Here's how the part is built. I have some questions about the finished solid (model axes, mm). A direction names the side the tool comes from. Coordinates: 2 decimals unless noted, no trailing zeros. Write each loop counter-clockwise with the first axis right and the second up, starting at its lowest first coordinate (ties: lowest second). Pieces come first, ordered by that corner, then holes. Notation, with made-up numbers: M -35,-27.5 L -14,-27.5 A25 ccw -14,3.5 Z; hole C 15.25,9.25 d8. An arc over 180 degrees is marked long. Use a Markdown table: item, result.
```python
from build123d import *

# Parameters (mm, degrees)
SKETCH1_W               = 111.06
SKETCH1_H               = 59.85
FACE_2_DEPTH            = 3.86
FACE_FILLETS_R          = 1
SKETCH2_W               = 106.25
SKETCH2_H               = 55.5
BODY_DEPTH              = 144
SKETCH3_W               = 12.75
SKETCH3_H               = 12.75
FEET_DEPTH              = 3.33
FEET_DRAFT              = 25
FEET_PROFILE_2_DEPTH    = 3.33
FEET_PROFILE_2_DRAFT    = 25
FEET_PROFILE_3_DEPTH    = 3.33
FEET_PROFILE_3_DRAFT    = 25
FEET_PROFILE_4_DEPTH    = 3.33
FEET_PROFILE_4_DRAFT    = 25
BODY_FILLETS_R          = 1
SKETCH4_R               = 5
GND_BANNANA_PORT_DEPTH  = 5.15
FILLET3_R               = 1
SKETCH5_W               = 50.3
SKETCH5_H               = 30.9
POWER_PORT_DEPTH        = 3.5
FILLET4_R               = 1
BOSS_EXTRUDE6_DEPTH     = 8.1
SKETCH7_R               = 6.5
BOSS_EXTRUDE7_DEPTH     = 2.35
SKETCH8_R               = 2.65
BOSS_EXTRUDE8_DEPTH     = 0.3
MIRROR2_COPY_1_SKETCH_R = 2.65
MIRROR2_COPY_1_DEPTH    = 0.3


with BuildPart() as part:
    # Sketch1 → Face 2 (new body)
    with BuildSketch(Plane.XY):
        Rectangle(SKETCH1_W, SKETCH1_H)
    extrude(amount=FACE_2_DEPTH)

    # Face Fillets
    face_fillets_edges = [part.edges().sort_by_distance(p)[0] for p in [
        (55.53, -29.925, 1.93),
        (-55.53, -29.925, 1.93),
        (-55.53, 29.925, 1.93),
        (55.53, 29.925, 1.93),
    ]]
    fillet(face_fillets_edges, radius=FACE_FILLETS_R)

    # Sketch2 → Body (add)
    with BuildSketch(Plane.XY):
        Rectangle(SKETCH2_W, SKETCH2_H)
    extrude(amount=BODY_DEPTH)


with BuildPart() as feet_tool:
    # Sketch3 → Feet (with draft: the straight prism first)
    with BuildSketch(Plane.XZ.offset(27.75)):
        with Locations((-36.625, 125.75)):
            Rectangle(SKETCH3_W, SKETCH3_H)
    extrude(amount=FEET_DEPTH)
    # Feet: the draft: its side faces are tilted about the plane it starts from
    feet_sides = [feet_tool.faces().sort_by_distance(p)[0] for p in [
        (-36.625, -29.415, 119.375),
        (-30.25, -29.415, 125.75),
        (-36.625, -29.415, 132.125),
        (-43, -29.415, 125.75),
    ]]
    draft(feet_sides, Plane.XZ.offset(27.75), FEET_DRAFT)


with BuildPart() as part_1:
    add(part.part)

    # Feet: add feet_tool
    add(feet_tool.part)


with BuildPart() as feet_profile_2_tool:
    # Sketch3 → Feet profile 2 (with draft: the straight prism first)
    with BuildSketch(Plane.XZ.offset(27.75)):
        with Locations((36.625, 125.75)):
            Rectangle(SKETCH3_W, SKETCH3_H)
    extrude(amount=FEET_PROFILE_2_DEPTH)
    # Feet profile 2: the draft: its side faces are tilted about the plane it starts from
    feet_profile_2_sides = [feet_profile_2_tool.faces().sort_by_distance(p)[0] for p in [
        (36.625, -29.415, 119.375),
        (43, -29.415, 125.75),
        (36.625, -29.415, 132.125),
        (30.25, -29.415, 125.75),
    ]]
    draft(feet_profile_2_sides, Plane.XZ.offset(27.75), FEET_PROFILE_2_DRAFT)


with BuildPart() as part_2:
    add(part_1.part)

    # Feet profile 2: add feet_profile_2_tool
    add(feet_profile_2_tool.part)


with BuildPart() as feet_profile_3_tool:
    # Sketch3 → Feet profile 3 (with draft: the straight prism first)
    with BuildSketch(Plane.XZ.offset(27.75)):
        with Locations((36.625, 18.86)):
            Rectangle(SKETCH3_W, SKETCH3_H)
    extrude(amount=FEET_PROFILE_3_DEPTH)
    # Feet profile 3: the draft: its side faces are tilted about the plane it starts from
    feet_profile_3_sides = [feet_profile_3_tool.faces().sort_by_distance(p)[0] for p in [
        (36.625, -29.415, 12.485),
        (43, -29.415, 18.86),
        (36.625, -29.415, 25.235),
        (30.25, -29.415, 18.86),
    ]]
    draft(feet_profile_3_sides, Plane.XZ.offset(27.75), FEET_PROFILE_3_DRAFT)


with BuildPart() as part_3:
    add(part_2.part)

    # Feet profile 3: add feet_profile_3_tool
    add(feet_profile_3_tool.part)


with BuildPart() as feet_profile_4_tool:
    # Sketch3 → Feet profile 4 (with draft: the straight prism first)
    with BuildSketch(Plane.XZ.offset(27.75)):
        with Locations((-36.625, 18.86)):
            Rectangle(SKETCH3_W, SKETCH3_H)
    extrude(amount=FEET_PROFILE_4_DEPTH)
    # Feet profile 4: the draft: its side faces are tilted about the plane it starts from
    feet_profile_4_sides = [feet_profile_4_tool.faces().sort_by_distance(p)[0] for p in [
        (-36.625, -29.415, 12.485),
        (-30.25, -29.415, 18.86),
        (-36.625, -29.415, 25.235),
        (-43, -29.415, 18.86),
    ]]
    draft(feet_profile_4_sides, Plane.XZ.offset(27.75), FEET_PROFILE_4_DRAFT)


with BuildPart() as part_4:
    add(part_3.part)

    # Feet profile 4: add feet_profile_4_tool
    add(feet_profile_4_tool.part)

    # Body Fillets
    body_fillets_edges = [part_4.edges().sort_by_distance(p)[0] for p in [
        (53.125, -27.75, 73.93),
        (53.125, 27.75, 73.93),
        (-53.125, 27.75, 73.93),
        (-53.125, -27.75, 73.93),
    ]]
    fillet(body_fillets_edges, radius=BODY_FILLETS_R)

    # Sketch4 → GND Bannana Port (add)
    with BuildSketch(Plane.XY.offset(144)):
        with Locations(Location((-33.825, 0, 0), (0, 0, 180))):
            Circle(SKETCH4_R)
    extrude(amount=GND_BANNANA_PORT_DEPTH)

    # Fillet3
    fillet3_edges = [part_4.edges().sort_by_distance(p)[0] for p in [
        (-28.825, 0, 149.15),
    ]]
    fillet(fillet3_edges, radius=FILLET3_R)

    # Sketch5 → Power Port (add)
    with BuildSketch(Plane.XY.offset(144)):
        with Locations((11.775, 0)):
            Rectangle(SKETCH5_W, SKETCH5_H)
    extrude(amount=POWER_PORT_DEPTH)

    # Fillet4
    fillet4_edges = [part_4.edges().sort_by_distance(p)[0] for p in [
        (36.925, -15.45, 145.75),
        (36.925, 15.45, 145.75),
        (-13.375, 15.45, 145.75),
        (-13.375, -15.45, 145.75),
    ]]
    fillet(fillet4_edges, radius=FILLET4_R)

    # Sketch6 → Boss-Extrude6 (add, symmetric)
    with BuildSketch(Plane(origin=(25, 0, 0), x_dir=(0, 0, -1), z_dir=(1, 0, 0))):
        with BuildLine():
            Line((-148.2, 13.502222039), (-148.2, 1.62259302))
            ThreePointArc((-148.2, 1.62259302), (-148.366278541, 0), (-148.858202027, -1.55514242))
            Line((-148.858202027, -1.55514242), (-153, -11.124297731))
            ThreePointArc((-153, -11.124297731), (-130.758589265, -2.678363494), (-148.2, 13.502222039))
        make_face()
    extrude(amount=BOSS_EXTRUDE6_DEPTH, both=True)

    # Sketch7 → Boss-Extrude7 (add, symmetric)
    with BuildSketch(Plane(origin=(0, 0, 0), x_dir=(-1, 0, 0), z_dir=(0, 0, -1))):
        with Locations((-34.53, -2.925)):
            Circle(SKETCH7_R)
    extrude(amount=BOSS_EXTRUDE7_DEPTH, both=True)

    # Sketch8 → Boss-Extrude8 (add, symmetric)
    with BuildSketch(Plane.XY.offset(144)):
        with Locations(Location((-47.825, 23.75, 0), (0, 0, 180))):
            Circle(SKETCH8_R)
    boss_extrude8 = extrude(amount=BOSS_EXTRUDE8_DEPTH, both=True)

    # Mirror1: Boss-Extrude8 across plane
    add(boss_extrude8.mirror(Plane(origin=(0, 0, 0), x_dir=(0, 0, 1), z_dir=(1, 0, 0))))

    # Mirror2: Boss-Extrude8 across plane
    add(boss_extrude8.mirror(Plane.ZX))

    # Mirror2 copy 1 sketch → Mirror2 copy 1 (add, symmetric)
    with BuildSketch(Plane(origin=(0, 0, 144), x_dir=(-1, 0, 0), z_dir=(0, 0, 1))):
        with Locations(Location((-47.825, 23.75, 0), (0, 0, 180))):
            Circle(MIRROR2_COPY_1_SKETCH_R)
    extrude(amount=MIRROR2_COPY_1_DEPTH, both=True)


solid = part_4.part
```
1. Suppose I cut it at D-D on y = 23.75. Write out the boundary of the cut face in (x, z) (3 decimals), and give its area (3 significant figures).
Answers follow:
| item | result |
|---|---|
| outline | M -55.53,0 L 55.53,0 L 55.53,3.86 L 53.125,3.86 L 53.125,144 L 50.475,144 L 50.475,144.3 L 45.175,144.3 L 45.175,144 L -45.175,144 L -45.175,144.3 L -50.475,144.3 L -50.475,144 L -53.125,144 L -53.125,3.86 L -55.53,3.86 Z |
| area | 15,300 mm2 |
2. Suppose I cut it at C-C on x = -5. Write out the boundary of the cut face in (y, z) (3 decimals), and give its area (3 significant figures).
Answers follow:
| item | result |
|---|---|
| outline | M -29.925,0 L 29.925,0 L 29.925,3.86 L 27.75,3.86 L 27.75,144 L 15.45,144 L 15.45,147.5 L -15.45,147.5 L -15.45,144 L -27.75,144 L -27.75,3.86 L -29.925,3.86 Z |
| area | 8,120 mm2 |
3. Suppose I cut it at A-A on y = -19. Write out the boundary of the cut face in (x, z) (3 decimals), and give its area (3 significant figures).
Answers follow:
| item | result |
|---|---|
| outline | M -55.53,0 L 55.53,0 L 55.53,3.86 L 53.125,3.86 L 53.125,144 L -53.125,144 L -53.125,3.86 L -55.53,3.86 Z |
| area | 15,300 mm2 |
4. Which directions (+Z, -Z, +X, -X, +Y, -Y) give clear straight access to the entire face, cutting with the end or side of a thin tool? Please do faces 1 (the face through (25.113, 0.022, 148.362)), 2 (the face through (-36.71, -29.39, 24.47)), 3 (the face through (-24, 0, 144)), 4 (the face through (28.33, -0.97, -1.19)), 5 (the face through (53.125, 0, 73)).
Answers follow:
| item | result |
|---|---|
| face 1 | +Z, +X, +Y |
| face 2 | +X, -X, -Y |
| face 3 | +Z |
| face 4 | -Z |
| face 5 | +Z, +X, +Y, -Y |
5. We'd pull the mould along Z, two halves only. Please class faces 6 (the face through (36.54, -29.39, 24.47)), 7 (the face through (-36.71, -29.39, 131.36)), 8 (the face through (-1, -29.925, 2)): +Z half, -Z half, draft (parallel to the pull), parting line (faces both ways), or undercut.
Answers follow:
| item | result |
|---|---|
| face 6 | undercut |
| face 7 | +Z half |
| face 8 | draft |
6. Suppose I cut it at B-B on z = 115. Write out the boundary of the cut face in (x, y) (3 decimals), and give its area (3 significant figures).
Answers follow:
| item | result |
|---|---|
| outline | M -53.125,-26.75 A1 ccw -52.125,-27.75 L 52.125,-27.75 A1 ccw 53.125,-26.75 L 53.125,26.75 A1 ccw 52.125,27.75 L -52.125,27.75 A1 ccw -53.125,26.75 Z |
| area | 5,900 mm2 |
7. Will these pins go through, and if not, where does the flat tip stop? pin 1 Ø1 at (x, z) = (-10.5, 37) entering from -Y; pin 2 Ø10 at (x, y) = (2.5, 11.5) entering from +Z; pin 3 Ø3 at (y, z) = (-24.5, 42.5) entering from -X (3 decimals).
Answers follow:
| item | result |
|---|---|
| pin 1 | stops at y = -27.75 |
| pin 2 | stops at z = 147.5 |
| pin 3 | stops at x = -53.125 |
8. I need wall thicknesses on probe 1 along Y at (x, z) = (23, 143); probe 2 along Z at (x, y) = (44.5, 23); probe 3 along X at (y, z) = (-19, 54) (3 decimals). Which ranges of each line are inside material? Lowest first, please.
Answers follow:
| item | result |
|---|---|
| probe 1 | y = -27.75 to 27.75 |
| probe 2 | z = 0 to 144 |
| probe 3 | x = -53.125 to 53.125 |
